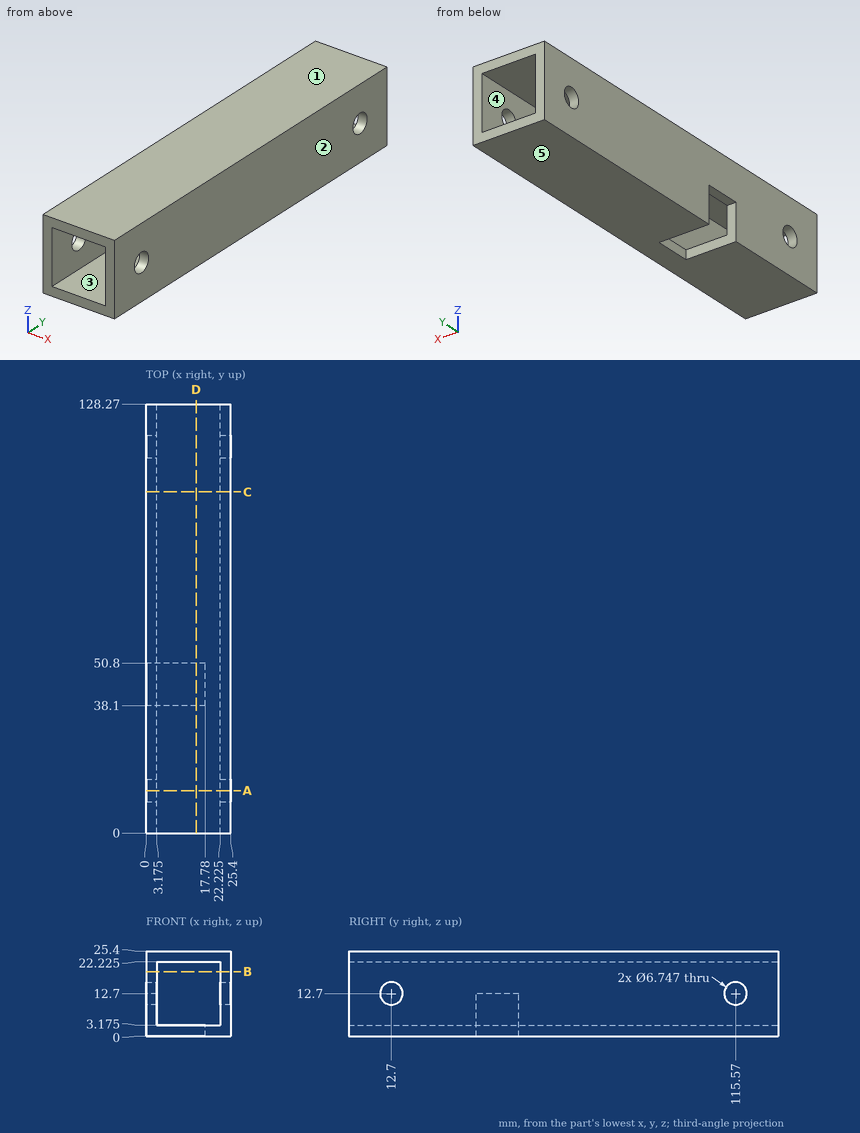
Design review of the part shown in the three views and the two pictorial views. Dimensions are in mm from the part's minimum x, y and z. A direction names the side the tool comes from. Round coordinates to 2 decimals unless told otherwise and drop trailing zeros. Write each loop counter-clockwise with the first axis right and the second up, starting at its lowest first coordinate (ties: lowest second). Pieces come first, ordered by that corner, then holes.
Item 1: We need section D-D on x = 15. Write out the cut boundary in (y, z) (3 decimals).
Item 2: For probe 1 along Y at (x, z) = (23.65, 12.7); probe 2 along X at (y, z) = (115, 5) (3 decimals), list the stretches that pass through material, from the lowest coordinate up.
Item 3: We need section B-B on z = 19.25. Write out the cut boundary in (x, y) (3 decimals).
Item 4: Clearance check with flat-ended pins moving along their axes: pin 1 Ø10 at (x, z) = (18, 3.5) entering from -Y; pin 2 Ø2 at (x, y) = (5.5, 47.5) entering from -Z (3 decimals); pin 3 Ø1.6 at (x, y) = (1, 46) entering from -Z; pin 4 Ø1.6 at (y, z) = (45, 1) entering from -X. State where each tip first meets the part, or that it passes through.
Item 5: The part is to be moulded in two halves that separate along Z. For the marked faces 1, 2 and 3, say which applies: +Z half, -Z half, draft (parallel to the pull), parting line (faces both ways), or undercut.
Item 6: For the marked faces 4 and 5, list the 3-axis set-ups (+Z, -Z, +X, -X, +Y, -Y) from which the entire face can be reached by the end or side of a thin tool; tool diameter is ignored.
Item 7: We need section C-C on y = 102. Write out the cut boundary in (x, z) (3 decimals), and give its area (3 significant figures).
Item 8: We need section A-A on y = 12.7. Write out the cut boundary in (x, z) (1 decimal).
Returned:
1. outline: (0, 0) - (38.1, 0) - (38.1, 3.175) - (0, 3.175) - close; (0, 22.225) - (128.27, 22.225) - (128.27, 25.4) - (0, 25.4) - close; (50.8, 0) - (128.27, 0) - (128.27, 3.175) - (50.8, 3.175) - close
2. probe 1: y = 0 to 9.33, 16.07 to 112.2, 118.94 to 128.27
2. probe 2: x = 0 to 3.175, 22.225 to 25.4
3. outline: (0, 0) - (3.175, 0) - (3.175, 128.27) - (0, 128.27) - close; (22.225, 0) - (25.4, 0) - (25.4, 128.27) - (22.225, 128.27) - close
4. pin 1: stops at y = 0
4. pin 2: stops at z = 22.225
4. pin 3: stops at z = 12.7
4. pin 4: stops at x = 17.78
5. face 1: +Z half
5. face 2: draft
5. face 3: undercut
6. face 4: +Y, -Y
6. face 5: -Z, +X, -X, +Y, -Y
7. outline: (0, 0) - (25.4, 0) - (25.4, 25.4) - (0, 25.4) - close; hole (3.175, 3.175) - (22.225, 3.175) - (22.225, 22.225) - (3.175, 22.225) - close
7. area: 282 mm2
8. outline: (0, 0) - (25.4, 0) - (25.4, 9.3) - (22.2, 9.3) - (22.2, 3.2) - (3.2, 3.2) - (3.2, 9.3) - (0, 9.3) - close; (0, 16.1) - (3.2, 16.1) - (3.2, 22.2) - (22.2, 22.2) - (22.2, 16.1) - (25.4, 16.1) - (25.4, 25.4) - (0, 25.4) - close
